Autodesk Inventor part; units mm, degrees
ref_plane "Work Plane2" through (0, -13.2935, -27.0771) normal (0, -0.988012, -0.1543769) x (-1, 0, 0)
ref_plane "YZ Plane" through (0, 0, 0) normal (1, 0, 0) x (0, 1, 0)
ref_plane "XZ Plane" through (0, 0, 0) normal (0, 1, 0) x (-1, 0, 0)
ref_plane "Work Plane1" through (0, 0, 1) normal (0, 0, 1) x (1, 0, 0)
sketch "Sketch2" plane through (0, 0, 1) normal (0, 0, 1) x (1, 0, 0)
  line L0 (-29.9972, 16.3668) -> (29.9972, 16.3668) construction
  line L1 (29.9972, -16.3668) -> (-29.9972, -16.3668) construction
  circle A0 centre (0, 0) radius 8 construction
  line L2 (-18, -2.183) -> (-18, 3.067) construction
  line L3 (17.5, -1.0311) -> (17.5, 1.567) construction
  line L4 (0, 16.3668) -> (0, 17.3668) construction
  line L5 (0, -16.3668) -> (0, -17.3668) construction
  line L6 (0, 17.3668) -> (-30, 17.3668) construction
  line L7 (0, 17.3668) -> (30, 17.3668) construction
  line L8 (-30, 17.3668) -> (30, 17.3668) construction
  line L9 (30, 17.3668) -> (30, -17.3668) construction
  line L10 (30, -17.3668) -> (-30, -17.3668) construction
  line L11 (-30, -17.3668) -> (-30, 17.3668) construction
  line L12 (-30, 17.3668) -> (-15, 17.3668)
  line L13 (-15, 17.3668) -> (-15, -17.3668)
  line L14 (-15, -17.3668) -> (-30, -17.3668)
  line L15 (-30, -17.3668) -> (-30, 17.3668)
  line L16 (30, 17.3668) -> (15, 17.3668)
  line L17 (15, 17.3668) -> (15, -17.3668)
  line L18 (15, -17.3668) -> (30, -17.3668)
  line L19 (30, -17.3668) -> (30, 17.3668)
  point P0 (0, 0)
  dimension "d0" = 1
  dimension "d1" = 1
  dimension "d2" = 30
  dimension "d3" = 30
  dimension "d4" = 15
  dimension "d5" = 15
extrude "Extrusion1" add sketch "Sketch2" along normal blind 5
ref_plane "Work Plane2" through (0, -13.2935, -27.0771) normal (0, -0.988012, -0.1543769) x (-1, 0, 0)
sketch "Sketch3" plane through (0, -13.2935, -27.0771) normal (0, -0.988012, -0.1543769) x (-1, 0, 0)
  line L0 (15, -28.3694) -> (30, -28.3694)
  line L1 (15, -28.3694) -> (15, -33.3094)
  line L2 (30, -33.3094) -> (15, -33.3094)
  line L3 (30, -28.3694) -> (30, -33.3094)
  line L4 (-15, -28.3694) -> (-30, -28.3694)
  line L5 (-30, -28.3694) -> (-30, -33.3094)
  line L6 (-15, -33.3094) -> (-30, -33.3094)
  line L7 (-15, -28.3694) -> (-15, -33.3094)
  line L8 (-24.9964, -11.75) -> (24.9964, -11.75)
  line L9 (-30, -33.3094) -> (30, -33.3094)
  line L10 (30, -33.3094) -> (30, -11.3094)
  line L11 (30, -11.3094) -> (-30, -11.3094)
  line L12 (-30, -11.3094) -> (-30, -33.3094)
  point P0 (0, -24.7003)
  dimension "d8" = 60
  dimension "d9" = 22
extrude "Extrusion2" add sketch "Sketch3" along normal blind 5
sketch "Sketch5" plane through (-30, -17.3668, 1) normal (-1, 0, 0) x (0, 0, 1)
  line L0 (0, 0) -> (0, 34.7337)
  line L1 (0, 0) -> (5, 0)
  line L2 (5, 34.7337) -> (5, 0)
  line L3 (0, 34.7337) -> (5, 34.7337)
  line L4 (4.833, -1.0688) -> (-16.9033, 2.3275)
  line L5 (-16.9033, 2.3275) -> (-17.6752, -2.6126)
  line L6 (4.0611, -6.0089) -> (-17.6752, -2.6126)
  line L7 (4.833, -1.0688) -> (4.0611, -6.0089)
  line L8 (5, 0) -> (5, -6.1556)
  line L9 (4.0611, -6.0089) -> (-17.6752, -2.6126)
  line L10 (5, -6.1556) -> (4.0611, -6.0089)
  line L11 (0, 0) -> (5, 0)
  line L12 (0, 0) -> (0, -3.0778)
  line L13 (4.833, -1.0688) -> (4.0611, -6.0089)
  line L14 (0, -3.0778) -> (4.0611, -6.0089)
  point P0 (-1, 17.3668)
extrude "Extrusion3" add sketch "Sketch5" against normal up to surface (60 mm away) contours L1 L8 L10 L7 L4 L12 | L4 L7 L14 L12
sketch "Sketch6" plane through (-30, 17.3668, 1) normal (-1, 0, 0) x (0, 0, 1)
  line L0 (0, -35.0474) -> (0, 0)
  line L1 (0, -35.0474) -> (-16.9033, -32.4062)
  line L2 (-16.9033, -32.4062) -> (-17.6752, -37.3463)
  line L3 (-17.6752, -37.3463) -> (5, -40.8893)
  line L4 (5, 0) -> (5, -40.8893)
  line L5 (0, 0) -> (5, 0)
  line L6 (-16.9033, -32.4062) -> (-24.0532, -32.4062)
  line L7 (-24.0532, -32.4062) -> (-24.0532, -41.4181)
  line L8 (-24.0532, -41.4181) -> (-16.9033, -41.4181)
  line L9 (-16.9033, -41.4181) -> (-16.9033, -32.4062)
  line L10 (-16.9033, -32.4062) -> (-14.9033, -32.4062)
  line L11 (-14.9033, -32.4062) -> (-14.9033, -41.4181)
  line L12 (-14.9033, -41.4181) -> (-16.9033, -41.4181)
  line L13 (-16.9033, -41.4181) -> (-16.9033, -32.4062)
  point P0 (-1, -17.3668)
  dimension "d18" = 2
extrude "Extrusion4" cut sketch "Sketch6" against normal through all contours L11 L3 L9 L1 | L1 L10 L11 | L9 L3 L2 | L2 L3 L9 L8 L7 L6 | L11 L12 L9 L3
sketch "Sketch7" plane through (-30, 17.3668, 1) normal (0, 1, 0) x (1, 0, 0)
  line L0 (0, 0) -> (15, 0)
  line L1 (0, 0) -> (0, -5)
  line L2 (15, -5) -> (0, -5)
  line L3 (15, 0) -> (15, -5)
  line L4 (60, 0) -> (45, 0)
  line L5 (45, 0) -> (45, -5)
  line L6 (60, -5) -> (45, -5)
  line L7 (60, 0) -> (60, -5)
  point P0 (30, 1)
extrude "Extrusion5" add sketch "Sketch7" along normal blind 5
ref_plane "Work Plane3" through (-30, -20.4125, -11.9033) normal (0, 0, -1) x (-1, 0, 0)
sketch "Sketch8" plane through (-30, -20.4125, -11.9033) normal (0, 0, -1) x (-1, 0, 0)
  line L0 (-7.7, 0) -> (-6, 0)
  line L1 (-2.3, 5.0607) -> (-7.7, 5.0607)
  circle A0 centre (-5, 2.5303) radius 1.5
  line L2 (-7.7, 0) -> (-6, 0)
  line L3 (-57.6, 0) -> (-52.4, 0)
  line L4 (-52.4, 0) -> (-52.4, -6.7313)
  line L5 (-52.4, -6.7313) -> (-57.6, -6.7313)
  line L6 (-57.6, -6.7313) -> (-57.6, 0)
  line L7 (-7.6, 1.0292) -> (-2.4, 1.0292)
  line L8 (-2.4, 1.0292) -> (-2.4, -4.6372)
  line L9 (-2.4, -4.6372) -> (-7.6, -4.6372)
  line L10 (-7.6, -4.6372) -> (-7.6, 1.0292)
  line L11 (-6, 0) -> (-2.3, 0)
  line L12 (-2.3, 5.0607) -> (-7.7, 5.0607)
  line L13 (-6, 0) -> (-2.3, 0)
  circle A1 centre (-5, 2.5303) radius 1.5
  line L14 (-7.7, 5.0607) -> (-7.7, 0)
  line L15 (-2.3, 0) -> (-2.3, 5.0607)
  line L16 (-7.7, 5.0607) -> (-7.7, 0)
  line L17 (-2.3, 0) -> (-2.3, 5.0607)
  point P0 (-30, 20.4125)
  point P1 (-7.2835, 0)
  point P2 (-2.4, 0)
  point P3 (-7.2835, 0.8465)
  point P4 (-7.6, 1.0292)
  point P5 (-7.6, 4.0314)
  point P6 (-5.8173, 5.0607)
  point P7 (-4.1827, 5.0607)
  point P8 (-2.4, 4.0314)
extrude "Extrusion6" [suppressed]
sketch "Sketch9" plane through (-30, -20.4125, -13.9033) normal (0, 0, -1) x (-1, 0, 0)
  circle A0 centre (-55, 2.5303) radius 1.5
  circle A1 centre (-5, 2.5303) radius 1.5
  point P0 (-30, 20.4125)
extrude "Extrusion7" cut sketch "Sketch9" against normal blind 8
sketch "Sketch10" plane through (0, 0, 1) normal (0, 0, -1) x (-1, 0, 0)
  line L0 (15, 22.3649) -> (15, 22.3668)
  line L1 (30, 22.3668) -> (30, 22.3649)
  line L2 (30, 22.3668) -> (15, 22.3668)
  line L3 (-30, 22.3649) -> (-30, 22.3668)
  line L4 (-15, 22.3668) -> (-15, 22.3649)
  line L5 (-15, 22.3668) -> (-30, 22.3668)
  line L6 (-15, 22.3668) -> (-30, 22.3668)
  line L7 (-30, 22.3668) -> (-30, 19.8668)
  line L8 (-30, 22.3668) -> (-30, -17.6805)
  line L9 (-30, 19.8668) -> (-22.5, 19.8668)
  line L10 (30, 22.3668) -> (30, 19.8668)
  line L11 (30, -17.6805) -> (30, 22.3668)
  line L12 (30, 19.8668) -> (22.5, 19.8668)
  circle A0 centre (-22.5, 19.8668) radius 1.5
  circle A1 centre (22.5, 19.8668) radius 1.5
  line L13 (15, 22.3649) -> (30, 22.3649)
  line L14 (-30, 22.3649) -> (-15, 22.3649)
  point P0 (0, 0)
  point P1 (30, 17.3668)
  point P2 (-30, 17.3668)
  dimension "d24" = 2.5
  dimension "d25" = 7.5
  dimension "d26" = 2.5
  dimension "d27" = 7.5
  dimension "d28" = 3
  dimension "d29" = 3
extrude "Extrusion8" cut sketch "Sketch10" against normal through all
sketch "Sketch11" plane through (-30, -20.4125, -13.9033) normal (0, 0, -1) x (-1, 0, 0)
  circle A0 centre (-55, 2.5303) radius 1.5
  circle A1 centre (-5, 2.5303) radius 1.5
  point P0 (-30, 20.4125)
extrude "Extrusion9" cut sketch "Sketch11" against normal through all
sketch "Sketch12" plane through (-30, -20.4125, -13.9033) normal (-1, 0, 0) x (0, 0, 1)
  line L0 (0, 5.0607) -> (0, 0)
  line L1 (0, 0) -> (19.9033, -3.1099)
  line L2 (19.9033, -3.1099) -> (19.9033, 42.7794)
  line L3 (14.9033, 42.7794) -> (19.9033, 42.7794)
  line L4 (14.9033, 2.732) -> (14.9033, 42.7794)
  line L5 (14.9033, 2.732) -> (0, 5.0607)
  line L6 (0, 5.0607) -> (0, 6.0607)
  line L7 (6.5941, 4.0303) -> (14.9033, 2.732)
  line L8 (0, 6.0607) -> (14.9033, 2.732)
  point P0 (13.9033, 20.4125)
  dimension "d34" = 1
extrude "Extrusion10" add sketch "Sketch12" against normal up to surface (60 mm away) contours L6 L8 L5
sketch "Sketch13" plane through (-30, -23.5224, 6) normal (-1, 0, 0) x (0, 0, 1)
  line L0 (-19.9033, 4.1402) -> (0, 4.1402)
  line L1 (-19.9033, 7.1402) -> (0, 7.1402)
  line L2 (-19.9033, 9.1706) -> (-19.9033, 3.1099) construction
  line L3 (-19.9033, 3.1099) -> (0, 0) construction
  line L4 (0, 0) -> (0, 45.8893) construction
  line L5 (-5, 45.8893) -> (0, 45.8893)
  line L6 (-5, 5.8419) -> (-5, 45.8893)
  line L7 (-5, 5.8419) -> (-19.9033, 9.1706)
  line L8 (-19.9033, 3.1099) -> (0, 3.1099)
  line L9 (0, 3.1099) -> (0, 0)
  line L10 (0, 0) -> (-19.9033, 0)
  line L11 (-19.9033, 0) -> (-19.9033, 3.1099)
  point P0 (-6, 23.5224)
extrude "Extrusion11" add sketch "Sketch13" against normal up to surface (60 mm away) contours L8 L9 L10 L11
fillet "Fillet1" radius 1 14 edges at (0, -23.5224, 6) (-22.5, 22.3668, 6) (22.5, 22.3668, 6) (-30, -0.5778, 6) (-15, 2.5, 6) (0, -17.3668, 6) (15, 2.5, 6) (30, -0.5778, 6) (-30, -23.5224, -3.9516) (30, -23.5224, -3.9516) (-30, 22.3668, 3.5) (-15, 22.3668, 3.5) (15, 22.3668, 3.5) (30, 22.3668, 3.5)
sketch "Sketch14" plane through (30, -14.3519, -13.9033) normal (0, 0, -1) x (-1, 0, 0)
  circle A0 centre (5, -3.5303) radius 1.5
  circle A1 centre (55, -3.5303) radius 1.5
  line L0 (60, -8.1706) -> (60, 0)
  line L1 (60, 0) -> (0, 0)
  line L2 (0, 0) -> (0, -8.1706)
  line L3 (59, -9.1706) -> (1, -9.1706)
  arc A2 (59, -9.1706) -> (60, -8.1706) centre (59, -8.1706) ccw
  arc A3 (0, -8.1706) -> (1, -9.1706) centre (1, -8.1706) ccw
  point P0 (30, 14.3519)
extrude "Extrusion12" cut sketch "Sketch14" against normal blind 8
sketch "Sketch15" plane through (-30, -17.6805, 1) normal (-1, 0, 0) x (0, 0, 1)
  line L0 (-6.9033, 1.5418) -> (-6.9033, -4.8419)
  line L1 (4, 39.0474) -> (4, -4.8419)
  line L2 (0, 0) -> (0, 39.0474)
  line L3 (0, 0) -> (-6.9033, 1.5418)
  line L4 (4, -5.8419) -> (-6.9033, -5.8419)
  line L5 (-6.9033, -5.8419) -> (-43.1083, -5.8419)
  line L6 (-43.1083, -5.8419) -> (-43.1083, 9.6282)
  line L7 (-43.1083, 9.6282) -> (-6.9033, 9.6282)
  line L8 (-6.9033, 9.6282) -> (-6.9033, -5.8419)
  line L9 (4, -4.8419) -> (-6.9033, -4.8419)
  line L10 (0, 39.0474) -> (4, 39.0474)
  point P0 (-1, 17.6805)
extrude "Extrusion13" cut sketch "Sketch15" against normal through all contours L0 L8 L5 L6 L7
properties part number "camera_holder"
Geometry: final body of the model. Coordinates: model frame, mm. A direction names the side the tool comes from. Give positions to 0.01 mm unless a question says otherwise; leave off trailing zeros. Order: outer loops, then holes, each group sorted by start corner. A loop starts at its lowest first (then second) coordinate and runs counter-clockwise, first axis right, second up. Notation, with made-up numbers: M 53,55.5 L 72,55.5 A22 ccw 72,79.5 Z; hole C 17,33.5 d1. An arc over 180 degrees is marked long. Answer as CSV lines item,"result". Start each with the question number.
1) Line query: line 1 (X direction, y = -18, z = -0.5); line 2 (Y direction, x = -25, z = 2.75); line 3 (X direction, y = 1, z = 2). Output: solid intervals per line, ascending. Write a range as from..to.
2) Cut plane B-B (y = 11). Output: boundary loops of the cut face in (x, z).
3) Cut plane D-D (z = -0.25). Output: boundary loops of the cut face in (x, y), then the cut area to 3 significant figures.
4) Mould query, pull axis X, two halves, no side actions, for faces 6 (the flat face through (30, -5, 2)), 7 (the flat face through (-30, -5, 2)), 8 (the flat face through (0, -20, -5.903)), 9 (the flat face through (24.98, -17.15, -2.4)). Classes: +X half, -X half, draft (parallel to the pull), parting line (faces both ways), or undercut.
5) Set-up query: faces 1 (the flat face through (0, -20, 6)), 2 (the flat face through (-25.02, -17.15, -2.4)), 3 (the flat face through (-0.4, -16.9, -2.5)), 4 (the cylindrical face through (24, 19.9, 3.5)), 5 (the flat face through (0, -17.367, 3)). Return all of +Z, -Z, +X, -X, +Y, -Y with unobstructed straight access to the full face (end or side cutting, diameter ignored); none if empty.
6) First-contact query: P1, Ø1, axis at x = 17, z = -1, coming from the +Y side; P2, Ø1.2, axis at x = 6, z = 2, coming from the +Y side. Flat tips, straight axial feed; report the tip coordinate or a pass-through.
7) Cut plane C-C (x = -3). Output: boundary loops of the cut face in (y, z).
Findings below:
1,line 1,"x = -30..-26.5, -23.5..23.5, 26.5..30"
1,line 2,"y = -23.52..-19.38, -16.38..22.37"
1,line 3,"x = -30..-15, 15..30"
2,outline,"M -30,1 L -15,1 L -15,5 A1 ccw -16,6 L -29,6 A1 ccw -30,5 Z; M 15,1 L 30,1 L 30,5 A1 ccw 29,6 L 16,6 A1 ccw 15,5 Z"
3,outline,"M -30,-22.52 A1 ccw -29,-23.52 L 29,-23.52 A1 ccw 30,-22.52 L 30,-17.4 L -30,-17.4 Z; hole M -26.45,-17.49 A1.5 ccw long -23.55,-17.49 Z; hole M 23.55,-17.49 A1.5 ccw long 26.45,-17.49 Z"
3,area,"357 mm²"
4,face 6,"+X half"
4,face 7,"-X half"
4,face 8,"draft"
4,face 9,"undercut"
5,face 1,"+Z, +X, -X, +Y, -Y"
5,face 2,"-Z"
5,face 3,"+X, -X, +Y"
5,face 4,"+Z, -Z"
5,face 5,"+Z, +Y"
6,P1,"stops at y = -17.12"
6,P2,"stops at y = -17.37"
7,outline,"M -23.52,-5.9 L -16.14,-5.9 L -17.68,1 L -17.37,1 L -17.37,5 A1 ccw -18.37,6 L -22.52,6 A1 ccw -23.52,5 Z"
